from build123d import *

# Parameters (mm, degrees)
BOSS_EXTRUDE1_DEPTH = 10
BOSS_EXTRUDE2_START = -10
BOSS_EXTRUDE2_DEPTH = 10


with BuildPart() as part:
    # Sketch1 → Boss-Extrude1 (new body)
    with BuildSketch(Plane(origin=(0, 0, 0), x_dir=(1, 0, 0), z_dir=(0, 1, 0))):
        with BuildLine():
            Line((-0.5, 68.548309499), (0.5, 68.548309499))
            ThreePointArc((0.5, 68.548309499), (1.914213562, 69.134095936), (2.5, 70.548309499))
            Line((2.5, 70.548309499), (2.5, 76.509166118))
            ThreePointArc((2.5, 76.509166118), (0, -76.55), (-2.5, 76.509166118))
            Line((-2.5, 76.509166118), (-2.5, 70.548309499))
            ThreePointArc((-2.5, 70.548309499), (-1.914213562, 69.134095936), (-0.5, 68.548309499))
        make_face()
        with BuildLine():
            Line((-4.498898253, 64.545545648), (4.504620523, 64.545545648))
            ThreePointArc((4.504620523, 64.545545648), (5.918834085, 65.131332086), (6.504620523, 66.545545648))
            Line((6.504620523, 66.545545648), (6.504620523, 70.035519058))
            ThreePointArc((6.504620523, 70.035519058), (7.178383305, 71.532547729), (8.745715364, 72.020934198))
            ThreePointArc((8.745715364, 72.020934198), (31.254364336, 65.472644745), (50.5, 52.08889037))
            Line((50.5, 52.08889037), (50.5, 43))
            Line((50.5, 43), (54.5, 43))
            Line((54.5, 43), (54.5, 39))
            Line((54.5, 39), (61.17599611, 39))
            ThreePointArc((61.17599611, 39), (72.55, 0), (61.17599611, -39))
            Line((61.17599611, -39), (54.5, -39))
            Line((54.5, -39), (54.5, -43))
            Line((54.5, -43), (50.5, -43))
            Line((50.5, -43), (50.5, -52.08889037))
            ThreePointArc((50.5, -52.08889037), (0, -72.55), (-50.5, -52.08889037))
            Line((-50.5, -52.08889037), (-50.5, -43))
            Line((-50.5, -43), (-54.5, -43))
            Line((-54.5, -43), (-54.5, -39))
            Line((-54.5, -39), (-61.17599611, -39))
            ThreePointArc((-61.17599611, -39), (-72.50088526, 0), (-61.17599611, 39))
            Line((-61.17599611, 39), (-54.5, 39))
            Line((-54.5, 39), (-54.5, 43))
            Line((-54.5, 43), (-50.5, 43))
            Line((-50.5, 43), (-50.5, 52.08889037))
            ThreePointArc((-50.5, 52.08889037), (-31.251689593, 65.473921507), (-8.739830875, 72.021648525))
            ThreePointArc((-8.739830875, 72.021648525), (-7.172599878, 71.533188183), (-6.498898253, 70.036213693))
            Line((-6.498898253, 70.036213693), (-6.498898253, 66.545545648))
            ThreePointArc((-6.498898253, 66.545545648), (-5.913111815, 65.131332086), (-4.498898253, 64.545545648))
        make_face(mode=Mode.SUBTRACT)
    extrude(amount=BOSS_EXTRUDE1_DEPTH)

    # Sketch2 → Boss-Extrude2 (add)
    with BuildSketch(Plane(origin=(0, 10, 0), x_dir=(1, 0, 0), z_dir=(0, 1, 0)).offset(BOSS_EXTRUDE2_START)):
        with BuildLine():
            ThreePointArc((2.5, 76.509166118), (0, -76.55), (-2.5, 76.509166118))
            Line((-2.5, 76.509166118), (-2.5, 76.959404883))
            ThreePointArc((-2.5, 76.959404883), (0, -77), (2.5, 76.959404883))
            Line((2.5, 76.959404883), (2.5, 76.509166118))
        make_face()
    extrude(amount=BOSS_EXTRUDE2_DEPTH)


solid = part.part
Design review of the part built by this model. Coordinates are the model's own, in mm. Round coordinates to 2 decimals unless told otherwise and drop trailing zeros. Write each loop counter-clockwise with the first axis right and the second up, starting at its lowest first coordinate (ties: lowest second). Pieces come first, ordered by that corner, then holes. Notation, with made-up numbers: (60, 85) -> (78, 85) arc R19 ccw to (78, 121) -> close; hole circle Ø3 at (-3.5, -21). An arc over 180 degrees is marked (long way). One line per question, with ' | ' between items.
(1) Wall thickness on line 1 (X direction, y = 7, z = 52.5); line 2 (X direction, y = 7.75, z = 12); line 3 (Z direction, x = 20.5, y = 0.5): over which ranges is each line inside the solid? List them lowest first. Write a range as [from, to].
Result sheet:
line 1: [-56.33, -50.07], [50.07, 56.33] | line 2: [-76.06, -71.51], [71.55, 76.06] | line 3: [-74.22, -69.59], [69.59, 74.22]
(2) Draft analysis for pull direction X (two halves, no side actions). For faces 1 (the cylindrical face through (-3.351, 4.93, 76.927)), 2 (the flat face through (-6, 10, -69)), 3 (the flat face through (52, 5, -43)), 4 (the flat face through (-6.499, 5, -68)), state which applies: released by +X, released by -X, zero draft, split by the parting line, or undercut.
Result sheet:
face 1: split by the parting line | face 2: zero draft | face 3: undercut | face 4: undercut
(3) Insertion check: P1, Ø2, axis at x = 53, y = 3, coming from the +Z side; P2, Ø1.2, axis at y = 5, z = 40, coming from the +X side; P3, Ø5.5, axis at x = -58, y = 4, coming from the +Z side. Each pin has a flat end and moves straight along its axis. Give the tip position at first contact, or say it passes through.
Result sheet:
P1: z = 56.79 | P2: x = 66.16 | P3: z = 53.63
(4) Take a section at A-A, the plane z = 0. State the section outline as (x, y) points.
Result sheet:
outline: (-77, 0) -> (-72.5, 0) -> (-72.5, 10) -> (-77, 10) -> close; (72.55, 0) -> (77, 0) -> (77, 10) -> (72.55, 10) -> close
(5) Take a section at B-B, the plane x = 31.5. State the section outline as (y, z) points.
Result sheet:
outline: (0, -70.26) -> (10, -70.26) -> (10, -65.35) -> (0, -65.35) -> close; (0, 65.35) -> (10, 65.35) -> (10, 70.26) -> (0, 70.26) -> close
